from build123d import *

# Parameters (mm, degrees)
SKETCH1_W             = 140.208
SKETCH1_H             = 38.1
BOSS_EXTRUDE1_DEPTH   = 3
SKETCH2_OUTSIDE_W     = 171.272
SKETCH2_OUTSIDE_H     = 69.164
CUT_EXTRUDE1_DEPTH    = 73.708137894
F_8_CLEARANCE_HOLE1_D = 4.3053
F_6_CLEARANCE_HOLE1_D = 3.6576
FILLET1_R             = 5.08


with BuildPart() as part:
    # Sketch1 → Boss-Extrude1 (new body)
    with BuildSketch(Plane(origin=(0, 0, 0), x_dir=(1, 0, 0), z_dir=(0, 1, 0))):
        Rectangle(SKETCH1_W, SKETCH1_H)
    extrude(amount=BOSS_EXTRUDE1_DEPTH)

    # Sketch2 outside → Cut-Extrude1 (cut, through all)
    with BuildSketch(Plane(origin=(0, 3, 0), x_dir=(1, 0, 0), z_dir=(0, 1, 0))):
        Rectangle(SKETCH2_OUTSIDE_W, SKETCH2_OUTSIDE_H)
        with BuildLine():
            Line((-59.286266177, -17.212411161), (-35.488230904, 6.35))
            Line((-35.488230904, 6.35), (35.488230904, 6.35))
            Line((35.488230904, 6.35), (59.286266177, -17.212411161))
            ThreePointArc((59.286266177, -17.212411161), (68.266411161, -17.167733823), (68.221733823, -8.187588839))
            Line((68.221733823, -8.187588839), (40.711769096, 19.05))
            Line((40.711769096, 19.05), (-40.711769096, 19.05))
            Line((-40.711769096, 19.05), (-68.221733823, -8.187588839))
            ThreePointArc((-68.221733823, -8.187588839), (-68.266411161, -17.167733823), (-59.286266177, -17.212411161))
        make_face(mode=Mode.SUBTRACT)
    extrude(amount=-CUT_EXTRUDE1_DEPTH, mode=Mode.SUBTRACT)

    # #8 Clearance Hole1 (through all)
    with Locations(Plane(origin=(0, 3, 0), x_dir=(1, 0, 0), z_dir=(0, 1, 0))):
        with Locations((-63.754, -12.7), (63.754, -12.7)):
            Hole(F_8_CLEARANCE_HOLE1_D / 2)

    # #6 Clearance Hole1 (through all)
    with Locations(Plane(origin=(0, 3, 0), x_dir=(1, 0, 0), z_dir=(0, 1, 0))):
        with Locations((-54.729177678, -3.764532354), (-45.704355355, 5.170935292), (-38.1, 12.7), (0, 12.7), (38.1, 12.7), (45.704355355, 5.170935292), (54.729177678, -3.764532354), (-25.4, 12.7), (-12.7, 12.7), (12.7, 12.7), (25.4, 12.7)):
            Hole(F_6_CLEARANCE_HOLE1_D / 2)

    # Fillet1
    fillet1_edges = [part.edges().sort_by_distance(p)[0] for p in [
        (-40.711769096, 1.5, -19.05),
        (40.711769096, 1.5, -19.05),
        (35.488230904, 1.5, -6.35),
        (-35.488230904, 1.5, -6.35),
    ]]
    fillet(fillet1_edges, radius=FILLET1_R)


solid = part.part
CAD build for the part. Positions are in the model's coordinates, mm. A direction names the side the tool comes from. Coordinates: 2 decimals unless noted, no trailing zeros. Write each loop counter-clockwise with the first axis right and the second up, starting at its lowest first coordinate (ties: lowest second). Pieces come first, ordered by that corner, then holes. Notation, with made-up numbers: M -27,36 L -8,36 A34 cw -8,66 Z; hole C 14.25,-7 d1. An arc over 180 degrees is marked long. Answer as a JSON object with one key per item and string values. Group by question number.
1) Saw through at A-A (x = 25.4). Write the cut outline in (y, z).
2) Wall check: line 1 (X direction, y = 1.8, z = 2.5); line 2 (Z direction, x = 25.4, y = 1.1); line 3 (X direction, y = 1.95, z = 4). Give the ranges that are in metal, low to high. Write a range as from..to.
3) Saw through at C-C (z = 12.7). Write the cut outline in (x, y).
4) Saw through at B-B (z = -2). Write the cut outline in (x, y).
5) Mould opens along Z. For faces 3 (the face through (-35.357, 1.479, -5.958)), 4 (the face through (40.53, 1.48, -18.68)), 5 (the face through (56.556, 1.479, 3.684)) say: +Z half, -Z half, draft (parallel to the pull), parting line (faces both ways), or undercut.
6) Saw through at D-D (y = 1.9). Give the number of separate pieces and of enclosed holes in the cut face, plus the area to 3 significant figures.
7) Pin check, flat tips, straight feed: pin 1 Ø2 at (x, z) = (45.7, -5.17) entering from +Y; pin 2 Ø1 at (y, z) = (0.5, -11) entering from +X. Stop position of each tip, or through.
8) Tool access for faces 1 (the face through (47.97, 1.52, 6.01)), 2 (the face through (-56.474, 1.479, 3.215)): list every direction of +Z, -Z, +X, -X, +Y, -Y with a clear straight run to the whole face (end or side of a thin tool).
Values follow:
{
 "1": {"outline": "M 0,-19.05 L 3,-19.05 L 3,-14.53 L 0,-14.53 Z; M 0,-10.87 L 3,-10.87 L 3,-6.35 L 0,-6.35 Z"},
 "2": {"line 1": "x = -62.48..-56.05, -53.41..-44.43, 44.43..53.41, 56.05..62.48", "line 2": "z = -19.05..-14.53, -10.87..-6.35", "line 3": "x = -63.99..-56.54, -52.92..-45.94, 45.94..52.92, 56.54..63.99"},
 "3": {"outline": "M -70.1,0 L -65.91,0 L -65.91,3 L -70.1,3 Z; M -61.6,0 L -54.73,0 L -54.73,3 L -61.6,3 Z; M 54.73,0 L 61.6,0 L 61.6,3 L 54.73,3 Z; M 65.91,0 L 70.1,0 L 70.1,3 L 65.91,3 Z"},
 "4": {"outline": "M -57.93,0 L -39.88,0 L -39.88,3 L -57.93,3 Z; M 39.88,0 L 57.93,0 L 57.93,3 L 39.88,3 Z"},
 "5": {"face 3": "+Z half", "face 4": "-Z half", "face 5": "undercut"},
 "6": {"separate pieces": "1", "enclosed holes": "13", "area": "1,870 mm2"},
 "7": {"pin 1": "passes through", "pin 2": "stops at x = 49.35"},
 "8": {"face 1": "+Z, +Y, -Y", "face 2": "+Y, -Y"}
}
